from build123d import *

# Parameters (mm, degrees)
SKETCH1_R           = 12.1412
BOSS_EXTRUDE1_DEPTH = 12.192
FILLET1_R           = 10.16
SKETCH3_R           = 14.224
BOSS_EXTRUDE2_DEPTH = 5.08
FILLET6_R           = 2.032
SKETCH8_R           = 15.121257553
BOSS_EXTRUDE3_DEPTH = 5.08
FILLET7_R           = 1.016
SKETCH9_W           = 0.127
SKETCH9_H           = 4.070962721
CUT_EXTRUDE1_DEPTH  = 0.254
SKETCH13_R          = 14.74025754
BOSS_EXTRUDE4_DEPTH = 1.6383
SKETCH14_R          = 17.526
BOSS_EXTRUDE5_DEPTH = 0.508
BOSS_EXTRUDE6_DEPTH = 2.54
SKETCH16_R          = 12.446
BOSS_EXTRUDE7_DEPTH = 16.51
SKETCH17_R          = 10.16
BOSS_EXTRUDE8_DEPTH = 13.716
FILLET8_R           = 2.032


with BuildPart() as part:
    # Sketch1 → Boss-Extrude1 (new body)
    with BuildSketch(Plane(origin=(0, 0, 0), x_dir=(1, 0, 0), z_dir=(0, 1, 0))):
        with Locations(Location((0, 0, 0), (0, 0, 90))):
            Circle(SKETCH1_R)
    extrude(amount=BOSS_EXTRUDE1_DEPTH)

    # Fillet1
    fillet1_edges = [part.edges().sort_by_distance(p)[0] for p in [
        (0, 12.192, 12.1412),
    ]]
    fillet(fillet1_edges, radius=FILLET1_R)

    # Sketch3 → Boss-Extrude2 (add)
    with BuildSketch(Plane.XZ):
        with Locations(Location((0, 0, 0), (0, 0, 270))):
            Circle(SKETCH3_R)
    extrude(amount=BOSS_EXTRUDE2_DEPTH)

    # Sketch4 → Cut-Revolve1 (revolve, cut)
    with BuildSketch(Plane(origin=(0, 0, 0), x_dir=(0, 0, -1), z_dir=(1, 0, 0))):
        Polygon((11.292993812, 6.096), (6.681516056, 11.039365263), (11.292993812, 11.039365263), align=None)
    revolve(axis=Axis((0, 0, 0), (0, 1, 0)), mode=Mode.SUBTRACT)

    # Sketch5 → Cut-Revolve2 (revolve, cut)
    with BuildSketch(Plane(origin=(0, 0, 0), x_dir=(0, 0, -1), z_dir=(1, 0, 0))):
        Polygon((12.1412, 2.032), (11.292993812, 6.096), (14.961110493, 2.032), align=None)
    revolve(axis=Axis((0, 0, 0), (0, 1, 0)), mode=Mode.SUBTRACT)

    # Sketch7 → Cut-Revolve3 (revolve, cut)
    with BuildSketch(Plane.XY, mode=Mode.PRIVATE) as cut_revolve3_sk:
        Polygon((-10.086523159, 7.389300203), (-11.857198071, 4.504575846), (-11.857198071, 7.389300203), align=None)
    revolve(cut_revolve3_sk.sketch.rotate(Axis((0, 0, 0), (0, 1, 0)), 270), axis=Axis((0, 0, 0), (0, 1, 0)), mode=Mode.SUBTRACT)

    # Fillet6
    fillet6_edges = [part.edges().sort_by_distance(p)[0] for p in [
        (0, 0, 14.224),
    ]]
    fillet(fillet6_edges, radius=FILLET6_R)

    # Sketch8 → Boss-Extrude3 (add)
    with BuildSketch(Plane.XZ.offset(5.08)):
        with Locations(Location((0, 0, 0), (0, 0, 270))):
            Circle(SKETCH8_R)
    extrude(amount=BOSS_EXTRUDE3_DEPTH)

    # Fillet7
    # the kernel refuses this fillet: 1.016 mm, written as the material it takes off along each edge
    with BuildSketch(Plane(origin=(0, -5.08, 0), x_dir=(0, 0, -1), z_dir=(-1, 0, 0))) as fillet7_piece_1:
        with BuildLine():
            CenterArc((14.105257553, 1.009037279), FILLET7_R, 276.711639073, 83.288360927)
            Line((14.224, 0), (14.226374849, -0.020180746))
            ThreePointArc((14.226374849, -0.020180746), (14.672628776, -0.02032), (15.121257553, -0.02032))
            Line((15.121257553, -0.02032), (15.141577553, 0))
            Line((15.141577553, 0), (15.141577553, 1.009037279))
            Line((15.141577553, 1.009037279), (15.121257553, 1.009037279))
        make_face()
    revolve(axis=Axis((0, -5.08, 0), (0, -1, 0)), mode=Mode.SUBTRACT)

    # Sketch9 → Cut-Extrude1 (cut)
    with BuildSketch(Plane(origin=(-15.24, 0, 0), x_dir=(0, 0, -1), z_dir=(1, 0, 0))):
        with Locations((-0.0635, -8.124518639)):
            Rectangle(SKETCH9_W, SKETCH9_H)
    extrude(amount=CUT_EXTRUDE1_DEPTH, mode=Mode.SUBTRACT)

    # Sketch13 → Boss-Extrude4 (add)
    with BuildSketch(Plane.XZ.offset(10.16)):
        with Locations(Location((0, 0, 0), (0, 0, 90))):
            Circle(SKETCH13_R)
    extrude(amount=BOSS_EXTRUDE4_DEPTH)

    # Sketch14 → Boss-Extrude5 (add)
    with BuildSketch(Plane.XZ.offset(11.7983)):
        with Locations(Location((0, 0, 0), (0, 0, 270))):
            Circle(SKETCH14_R)
    extrude(amount=BOSS_EXTRUDE5_DEPTH)

    # Sketch15 → Boss-Extrude6 (add)
    with BuildSketch(Plane.XZ.offset(12.3063)):
        Polygon((15.24, 7.62), (15.24, -7.597992884), (0, -17.526), (-15.24, -7.597992884), (-15.24, 7.62), (0, 17.526), align=None)
    extrude(amount=BOSS_EXTRUDE6_DEPTH)

    # Sketch16 → Boss-Extrude7 (add)
    with BuildSketch(Plane.XZ.offset(14.8463)):
        with Locations(Location((0, 0, 0), (0, 0, 270))):
            Circle(SKETCH16_R)
    extrude(amount=BOSS_EXTRUDE7_DEPTH)

    # Sketch17 → Boss-Extrude8 (add)
    with BuildSketch(Plane.XZ.offset(31.3563)):
        with Locations(Location((0, 0, 0), (0, 0, 270))):
            Circle(SKETCH17_R)
    extrude(amount=BOSS_EXTRUDE8_DEPTH)

    # Fillet8
    fillet8_edges = [part.edges().sort_by_distance(p)[0] for p in [
        (0, -31.3563, 12.446),
    ]]
    fillet(fillet8_edges, radius=FILLET8_R)


solid = part.part
Can you work these out from the model? Positions are in its coordinate system, mm. A direction names the side the tool comes from. Coordinates: 2 decimals unless noted, no trailing zeros. Order: outer loops, then holes, each group sorted by start corner. A loop starts at its lowest first (then second) coordinate and runs counter-clockwise, first axis right, second up. Notation, with made-up numbers: M 40.5,16.5 L 66.5,16.5 A11 ccw 66.5,30.5 Z; hole C 6,44 d10. An arc over 180 degrees is marked long. Answer as CSV lines item,"result".
(1) Suppose I cut it at A-A on y = -27. Please give me the cut outline in (x, z).
Geometry check:
outline,"C 0,0 d24.89"
(2) I'm going to push flat-ended pins straight in: pin 1 (6 mm diameter, centred on x = 6, z = 9.5, fed in from +Y); pin 2 (1 mm diameter, centred on y = -4, z = -3, fed in from -X); pin 3 (1 mm diameter, centred on y = -18, z = -7, fed in from -X); pin 4 (5.5 mm diameter, centred on x = -10, z = -4, fed in from -Y). Where does each tip first touch, or does it pass through?
Geometry check:
pin 1,"y = 9.37"
pin 2,"x = -14"
pin 3,"x = -10.61"
pin 4,"y = -45.07"
(3) Please list where these lines run through material, in increasing order: L1, parallel to Y at x = -15, z = -6; L2, parallel to Y at x = 11.5, z = 12.5; L3, parallel to Z at x = 7, y = -29.5.
Geometry check:
L1,"-14.85 to -11.8"
L2,"-12.31 to -11.8"
L3,"-10.28 to 10.28"
(4) On a 3-axis mill with a long thin cutter (end or side, diameter ignored), from which of +Z, -Z, +X, -X, +Y, -Y can I reach the whole of each face in a straight line? I mean faces 1 (the cylindrical face through (7.388, 1.002, 9.635)), 2 (the flat face through (7.73, -13.56, -12.49)), 3 (the flat face through (16, -12.306, 3)), 4 (the flat face through (-7.73, -13.56, 12.5)), 5 (the flat face through (7.513, -13.559, 12.642)). Say none if no direction works.
Geometry check:
face 1,"+Y"
face 2,"-Z, +X, -Y"
face 3,"+X, -Y"
face 4,"+Z, -X, -Y"
face 5,"+Z, +X, -Y"
(5) If we mould it in two halves opening along Y, with no side actions, what happens to faces 6 (the cylindrical face through (10.074, -38.118, 1.323)), 7 (the flat face through (-6.6, -10.16, -13.4)), 8 (the flat face through (5, -14.846, -12))? For each: released by +Y, released by -Y, zero draft, split by the parting line, or undercut.
Geometry check:
face 6,"zero draft"
face 7,"undercut"
face 8,"released by -Y"
